```python
from build123d import *

# Parameters (mm, degrees)
F0_W     = 50.8
F0_H     = 50.8
F1_DEPTH = 50.8
F2_T     = -1.5875
F3_W     = 47.625
F3_H     = 0.79375
F4_DEPTH = 5.08
F7_DEPTH = 0.79375


# Not quite as in the source:
# - a length typed as a fraction of an inch, garbled in the dataset ("3 / 203.2 mm" for 3/8 in), is restored


with BuildPart() as f1:
    # F0 (on Right) → F1 (new body)
    with BuildSketch(Plane.YZ):
        with Locations((-4.0118778124, 15.742687114)):
            Rectangle(F0_W, F0_H)
    extrude(amount=F1_DEPTH)

    # F2
    f2_openings = [f1.faces().sort_by_distance(p)[0] for p in [
        (25.4, -4.011878, -9.657313),
    ]]
    offset(amount=F2_T, openings=f2_openings)

    # F3 (on face) → F4 (cut)
    with BuildSketch(Plane(origin=(0, 21.3881221876, 0), x_dir=(-1, 0, 0), z_dir=(0, 1, 0))):
        with Locations((-25.4, -9.260437886)):
            Rectangle(F3_W, F3_H)
    extrude(amount=-F4_DEPTH, mode=Mode.SUBTRACT)


with BuildPart() as f5_1:
    # F5: copy of F1
    add(f1.part)


with BuildPart() as f1_1:
    add(f1.part)

    # F7 (add): faces of the model
    f7_faces = [f1_1.faces().sort_by_distance(p)[0] for p in [
        (0.7184204897, -4.0118778124, -9.657312886),
        (25.4, 20.5943721876, -8.863562886),
    ]]
    extrude(f7_faces, amount=F7_DEPTH)


solid = f1_1.part
```
Can you work these out from the model? Positions are in its coordinate system, mm. A direction names the side the tool comes from. Coordinates: 2 decimals unless noted, no trailing zeros. Write each loop counter-clockwise with the first axis right and the second up, starting at its lowest first coordinate (ties: lowest second). Pieces come first, ordered by that corner, then holes. Notation, with made-up numbers: M -24,51 L -19,51 A28 ccw -19,71 Z; hole C -15.75,37 d4. An arc over 180 degrees is marked long. Write item = value, one per line. Start each with the question number.
Q1. On a 3-axis mill with a long thin cutter (end or side, diameter ignored), from which of +Z, -Z, +X, -X, +Y, -Y can I reach the whole of each face in a straight line? I mean faces 1 (the face through (25, -4, 39.555)), 2 (the face through (26, 21, -9.657)), 3 (the face through (0, -4, 16)). Say none if no direction works.
Q2. If we section it at A-A, the plane z = 5.5: Write out the boundary of the cut face in (x, y).
Q3. If we section it at C-C, the plane y = 1: Write out the boundary of the cut face in (x, z), then the cut area to 3 significant figures.
Q4. Thinking about a two-plate mould opening in X: for faces 4 (the face through (25, 19.801, 15)), 5 (the face through (25, -29.412, 16)), 6 (the face through (50.8, -4, 16)), which applies, released by +X, released by -X, zero draft, split by the parting line, or undercut?
Q5. If I drill on L1, parallel to X at y = -27, z = 31; L2, parallel to Y at x = 43, z = 27; L3, parallel to Z at x = 37, y = -14, over which ranges is the centre line in solid material (lowest first)? Write a range as [from, to].
Q6. I'm going to push flat-ended pins straight in: pin 1 (8 mm diameter, centred on x = 26.5, y = 9.5, fed in from -Z); pin 2 (1.7 mm diameter, centred on x = 22, y = 21, fed in from -Z). Where does each tip first touch, or does it pass through?
Q7. If we section it at B-B, the plane x = 18: Write out the boundary of the cut face in (y, z), then the cut area to 3 significant figures.
Check sheet entries:
q1.face_1 = -Z
q1.face_2 = -Z, +Y
q1.face_3 = +Z, -Z, -X, +Y, -Y
q2.outline = M 0,-29.41 L 50.8,-29.41 L 50.8,21.39 L 0,21.39 Z; hole M 1.59,-27.82 L 49.21,-27.82 L 49.21,19.8 L 1.59,19.8 Z
q3.outline = M 0,-10.45 L 1.59,-10.45 L 1.59,39.56 L 49.21,39.56 L 49.21,-10.45 L 50.8,-10.45 L 50.8,41.14 L 0,41.14 Z
q3.area = 239 mm²
q4.face_4 = undercut
q4.face_5 = zero draft
q4.face_6 = released by +X
q5.L1 = [0, 1.59], [49.21, 50.8]
q5.L2 = [-29.41, -27.82], [19.8, 21.39]
q5.L3 = [39.56, 41.14]
q6.pin_1 = 39.56
q6.pin_2 = -9.66
q7.outline = M -29.41,-10.45 L -27.82,-10.45 L -27.82,39.56 L 19.8,39.56 L 19.8,-9.66 L 21.39,-9.66 L 21.39,41.14 L -29.41,41.14 Z
q7.area = 238 mm²
